Autodesk Inventor part; units mm, degrees
ref_plane "YZ Plane" through (0, 0, 0) normal (1, 0, 0) x (0, 1, 0)
ref_plane "XZ Plane" through (0, 0, 0) normal (0, 1, 0) x (-1, 0, 0)
ref_plane "XY Plane" through (0, 0, 0) normal (0, 0, 1) x (1, 0, 0)
sketch "Boceto1" plane through (0, 0, 0) normal (0, 1, 0) x (-1, 0, 0)
  line L0 (0, -6.4663) -> (-5.6, -3.2332)
  line L1 (-5.6, -3.2332) -> (-5.6, 3.2332)
  line L2 (-5.6, 3.2332) -> (0, 6.4663)
  line L3 (0, 6.4663) -> (5.6, 3.2332)
  line L4 (5.6, 3.2332) -> (5.6, -3.2332)
  line L5 (5.6, -3.2332) -> (0, -6.4663)
  circle A0 centre (0, 0) radius 3.175
  line L6 (11, 0) -> (-11, 0) construction
  point P0 (2.8, -4.8497)
  point P1 (1.5875, -2.7496)
  point P2 (5.6, 0)
  dimension "d0" = 6.35
  dimension "d2" = 1.5875
  dimension "d4" = 22
  dimension "d10" = 11.2
extrude "Extrusión1" add sketch "Boceto1" along normal blind 5.55
thread "Rosca1"
chamfer "Chaflán1" distance 1 angle 45 12 edges at (-2.8, 5.55, 4.8497) (2.8, 5.55, 4.8497) (5.6, 5.55, 0) (2.8, 5.55, -4.8497) (-2.8, 5.55, -4.8497) (-5.6, 5.55, 0) (-5.6, 0, 0) (-2.8, 0, -4.8497) (2.8, 0, -4.8497) (5.6, 0, 0) (2.8, 0, 4.8497) (-2.8, 0, 4.8497)
properties part number "Tuerca1-4"
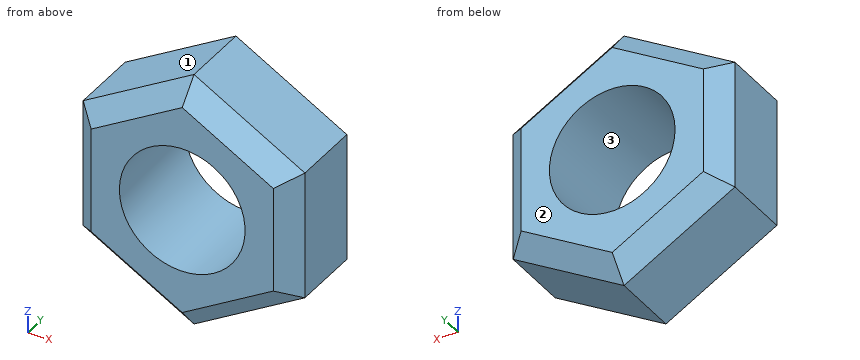
For this review, take the finished solid that the model builds, in its own axes (mm). Face numbers are marked on the shaded views. Coordinates: 2 decimals unless noted, no trailing zeros. Loops run counter-clockwise (first coordinate to the right, second up) from the corner with the lowest first, then second, coordinate; pieces in that order, holes last. Notation, with made-up numbers: (-35, -19) - (11, -19) arc R13 ccw to (11, 3) - close; hole circle Ø6 at (47, -40). An arc over 180 degrees is marked (long way). Use one line per item in the form item = value. Start each with the question number.
1) To check wall thickness, follow probe 1 along X at (y, z) = (0.35, 1.25); probe 2 along Z at (x, y) = (-1, 3.2); probe 3 along Z at (x, y) = (-1.75, 4.3). State the ranges of each line that lie inside material, in increasing order. Write a range as from..to.
2) Take a section at A-A (y = 2.75). State the section outline as (x, z) points (3 decimals).
3) Draft analysis for pull direction Z (two halves, no side actions). For the marked faces 1, 2 and 3, state which applies: released by +Z, released by -Z, zero draft, split by the parting line, or undercut.
4) Take a section at C-C (z = 0). State the section outline as (x, y) points (3 decimals).
5) Take a section at B-B (x = 2.75). State the section outline as (y, z) points, plus the area to 3 significant figures.
6) Take a section at D-D (z = 4.5). State the section outline as (x, y) points.
7) For pin 1 (3 mm diameter, centred on y = 4, z = -3.5, fed in from -X); pin 2 (5 mm diameter, centred on x = 0, z = 0, fed in from -Y), all flat-tipped, find the tip position at first contact; note any pin that passes through.
From the geometry:
q1.probe_1 = -4.95..-2.92, 2.92..4.95
q1.probe_2 = -5.89..-3.01, 3.01..5.89
q1.probe_3 = -5.46..-2.65, 2.65..5.46
q2.outline = (-5.6, -3.233) - (0, -6.466) - (5.6, -3.233) - (5.6, 3.233) - (0, 6.466) - (-5.6, 3.233) - close; hole circle Ø6.35 at (0, 0)
q3.face_1 = released by +Z
q3.face_2 = zero draft
q3.face_3 = undercut
q4.outline = (-5.6, 1) - (-4.6, 0) - (-3.175, 0) - (-3.175, 5.55) - (-4.6, 5.55) - (-5.6, 4.55) - close; (3.175, 0) - (4.6, 0) - (5.6, 1) - (5.6, 4.55) - (4.6, 5.55) - (3.175, 5.55) - close
q5.outline = (0, -3.72) - (1, -4.88) - (4.55, -4.88) - (5.55, -3.72) - (5.55, -1.59) - (0, -1.59) - close; (0, 1.59) - (5.55, 1.59) - (5.55, 3.72) - (4.55, 4.88) - (1, 4.88) - (0, 3.72) - close
q5.area = 34.2 mm2
q6.outline = (-3.41, 1) - (-1.41, 0) - (1.41, 0) - (3.41, 1) - (3.41, 4.55) - (1.41, 5.55) - (-1.41, 5.55) - (-3.41, 4.55) - close
q7.pin_1 = -5.6
q7.pin_2 = through
